CAD build for the part. Positions are in the model's coordinates, mm. A direction names the side the tool comes from. Round coordinates to 2 decimals unless told otherwise and drop trailing zeros. Order: outer loops, then holes, each group sorted by start corner. A loop starts at its lowest first (then second) coordinate and runs counter-clockwise, first axis right, second up. Notation, with made-up numbers: (76, 30.5) -> (94, 30.5) arc R6 ccw to (94, 39.5) -> close; hole circle Ø7 at (-18, 77). An arc over 180 degrees is marked (long way). Answer as CSV lines item,"result". Start each with the question number.
from build123d import *

# Parameters (mm, degrees)
BASE_FLANGE1_DEPTH           = 762
EDGE_FLANGE1_STRIP_W         = 28.3464
EDGE_FLANGE1_STRIP_H         = 0.7366
EDGE_FLANGE1_STRIP_CUT_DEPTH = 762
EDGE_FLANGE1_DEPTH           = 762
SKETCH9_R                    = 20.955
SKETCH9_W                    = 16.002
SKETCH9_H                    = 16.002
BOSS_EXTRUDE2_DEPTH          = 12.7


# Sheet-metal steps are written as plain solids
with BuildPart() as part:
    # Sketch3 → Base-Flange1 (new body)
    with BuildSketch(Plane.XY):
        with BuildLine():
            Line((-555.625, 0), (142.1384, 0))
            ThreePointArc((142.1384, 0), (151.639510976, -3.935489024), (155.575, -13.4366))
            Line((155.575, -13.4366), (155.575, -50.8))
            Line((155.575, -50.8), (154.8384, -50.8))
            Line((154.8384, -50.8), (154.8384, -13.4366))
            ThreePointArc((154.8384, -13.4366), (151.118656121, -4.456343879), (142.1384, -0.7366))
            Line((142.1384, -0.7366), (-555.625, -0.7366))
            Line((-555.625, -0.7366), (-555.625, 0))
        make_face()
    extrude(amount=BASE_FLANGE1_DEPTH)

    # Edge-Flange1 strip (across the edge) → Edge-Flange1 strip cut (cut)
    with BuildSketch(Plane(origin=(-555.625, -0.7366, 762), x_dir=(1, 0, 0), z_dir=(0, 0, -1))):
        with Locations((-0.7366, -0.3683)):
            Rectangle(EDGE_FLANGE1_STRIP_W, EDGE_FLANGE1_STRIP_H)
    extrude(amount=EDGE_FLANGE1_STRIP_CUT_DEPTH, mode=Mode.SUBTRACT)

    # Edge-Flange1 section (across the edge) → Edge-Flange1 (add)
    with BuildSketch(Plane(origin=(-555.625, -0.7366, 762), x_dir=(1, 0, 0), z_dir=(0, 0, -1))):
        with BuildLine():
            Line((0, 12.7), (0, 58.1914))
            Line((0, 58.1914), (0.7366, 58.1914))
            Line((0.7366, 58.1914), (0.7366, 12.7))
            ThreePointArc((0.7366, 12.7), (4.456343879, 3.719743879), (13.4366, 0))
            Line((13.4366, 0), (13.4366, -0.7366))
            ThreePointArc((13.4366, -0.7366), (3.935489024, 3.198889024), (0, 12.7))
        make_face()
    extrude(amount=EDGE_FLANGE1_DEPTH)

    # Sketch9 → Boss-Extrude2 (add)
    with BuildSketch(Plane(origin=(0, 0, 0), x_dir=(1, 0, 0), z_dir=(0, 1, 0))):
        with Locations(Location((-200.025, -381, 0), (0, 0, 270))):
            Circle(SKETCH9_R)
        with Locations((-200.025, -736.6)):
            Rectangle(SKETCH9_W, SKETCH9_H)
        with Locations((-200.025, -25.4)):
            Rectangle(SKETCH9_W, SKETCH9_H)
    extrude(amount=BOSS_EXTRUDE2_DEPTH)


solid = part.part
Item 1: Band-saw the part on A-A, the plane y = -38. Give the cut face in (x, z) (3 decimals).
Item 2: Band-saw the part on B-B, the plane z = 381. Give the cut face in (x, y) (3 decimals).
Item 3: Tool access for faces 3 (the flat face through (-200, 12.7, 381)), 4 (the flat face through (-195, -0.737, 376)): list every direction of +Z, -Z, +X, -X, +Y, -Y with a clear straight run to the whole face (end or side of a thin tool).
Item 4: Probe line 1 (X direction, y = -38.5, z = 693.5) (3 decimals); line 2 (Y direction, x = -503, z = 698); line 3 (X direction, y = -5.5, z = 33). List the from-to ranges inside material, lowest first.
Item 5: Band-saw the part on C-C, the plane x = -358. Give the cut face in (y, z).
Item 6: Band-saw the part on D-D, the plane z = 538. Give the cut face in (x, y) (3 decimals), and give its area (3 significant figures).
Item 7: Pin check, flat tips, straight feed: pin 1 (0.8 mm diameter, centred on x = 155, z = 237, fed in from -Y); pin 2 (14 mm diameter, centred on y = 6, z = 734, fed in from +X) (3 decimals); pin 3 (2 mm diameter, centred on y = -6.5, z = 270, fed in from +X). Stop position of each tip, or through.
Item 8: Mould opens along Z. For faces 1 (the flat face through (-200, 12.7, 736)), 2 (the cylindrical face through (-218.6, 6.3, 390.7)) say: released by +Z, released by -Z, zero draft, split by the parting line, or undercut.
Values:
1,outline,"(-555.625, 0) -> (-554.888, 0) -> (-554.888, 762) -> (-555.625, 762) -> close; (154.838, 0) -> (155.575, 0) -> (155.575, 762) -> (154.838, 762) -> close"
2,outline,"(-555.625, -58.928) -> (-554.888, -58.928) -> (-554.888, -13.437) arc R12.7 cw to (-542.188, -0.737) -> (142.138, -0.737) arc R12.7 cw to (154.838, -13.437) -> (154.838, -50.8) -> (155.575, -50.8) -> (155.575, -13.437) arc R13.437 ccw to (142.138, 0) -> (-179.07, 0) -> (-179.07, 12.7) -> (-220.98, 12.7) -> (-220.98, 0) -> (-542.188, 0) arc R13.437 ccw to (-555.625, -13.437) -> close"
3,face 3,"+Z, -Z, +X, -X, +Y"
3,face 4,"+Z, -Z, -Y"
4,line 1,"-555.625 to -554.888, 154.838 to 155.575"
4,line 2,"-0.74 to 0"
4,line 3,"-553.03 to -552.1, 152.05 to 152.98"
5,outline,"(-0.74, 0) -> (0, 0) -> (0, 762) -> (-0.74, 762) -> close"
6,outline,"(-555.625, -58.928) -> (-554.888, -58.928) -> (-554.888, -13.437) arc R12.7 cw to (-542.188, -0.737) -> (142.138, -0.737) arc R12.7 cw to (154.838, -13.437) -> (154.838, -50.8) -> (155.575, -50.8) -> (155.575, -13.437) arc R13.437 ccw to (142.138, 0) -> (-542.188, 0) arc R13.437 ccw to (-555.625, -13.437) -> close"
6,area,"595 mm²"
7,pin 1,"y = -50.8"
7,pin 2,"x = 147.225"
7,pin 3,"x = 154.19"
8,face 1,"zero draft"
8,face 2,"undercut"
